Geometry: final body of the model. Coordinates: model frame, mm. Coordinates: 2 decimals unless noted, no trailing zeros. Order: outer loops, then holes, each group sorted by start corner. A loop starts at its lowest first (then second) coordinate and runs counter-clockwise, first axis right, second up. Notation, with made-up numbers: (5.5, 77.25) - (31.5, 77.25) arc R21 ccw to (31.5, 95.25) - close; hole circle Ø3 at (23.5, 72.25). An arc over 180 degrees is marked (long way). Use a Markdown table: item, result. Add a question column.
```python
from build123d import *

# Parameters (mm, degrees)
DOME1_FACE_RADIUS = 41.275
DOME1_HEIGHT      = 9.525
FILLET1_R         = 2.54


# Read off the part's stored shape, not the designer's step: Shell1
with BuildPart() as part:
    # Sketch1 → Revolve1 (revolve)
    with BuildSketch(Plane(origin=(0, 0, 0), x_dir=(0, 0, -1), z_dir=(1, 0, 0)), mode=Mode.PRIVATE) as revolve1_sk:
        Polygon((0, 0), (41.275, 0), (43.78974535, 19.05), (0, 19.05), align=None)
    revolve(revolve1_sk.sketch.rotate(Axis((0, 0, 0), (0, -1, 0)), 180), axis=Axis((0, 0, 0), (0, -1, 0)))

    # Dome1: a dome of height H over a round flat face of radius A is a cap of a sphere of radius (A * A + H * H) / (2 * H)
    dome1_r = (DOME1_FACE_RADIUS * DOME1_FACE_RADIUS + DOME1_HEIGHT * DOME1_HEIGHT) / (2 * DOME1_HEIGHT)
    dome1_base = Plane((0, 0, 0), z_dir=(0, -1, 0))
    with Locations(dome1_base.offset(DOME1_HEIGHT - dome1_r)):
        dome1_ball = Sphere(dome1_r, mode=Mode.PRIVATE)
    add(split(dome1_ball, bisect_by=dome1_base, keep=Keep.TOP, mode=Mode.PRIVATE))

    # Fillet1
    fillet1_edges = [part.edges().sort_by_distance(p)[0] for p in [
        (41.275, 0, 0),
    ]]
    fillet(fillet1_edges, radius=FILLET1_R)

    # Shell1 outline → Shell1 (revolve, cut)
    with BuildSketch(Plane.XY):
        with BuildLine():
            Line((0, 19.05), (0, -6.35))
            ThreePointArc((0, -6.35), (19.639142672, -4.205925769), (38.353009101, 2.125281265))
            Line((38.353009101, 2.125281265), (40.587201031, 19.05))
            Line((40.587201031, 19.05), (0, 19.05))
        make_face()
    revolve(axis=Axis((0, 0, 0), (0, 1, 0)), mode=Mode.SUBTRACT)


solid = part.part
```
1) Section B-B (y = 17). Return loops of the section in (x, z).
2) Pin query (flat end, axial travel): pin 1 (5 mm diameter, centred on x = -33.5, y = 9.5, fed in from +Z); pin 2 (8 mm diameter, centred on x = -30, y = 2.5, fed in from -Z); pin 3 (10 mm diameter, centred on x = -34.5, z = -11.5, fed in from -Y). Return the tip coordinate at first contact, or that it passes through.
3) Section A-A (y = 12.5). Return loops of the section in (x, z), then the cut area to 3 significant figures.
4) Ray query, line 1 along X through (y, z) = (2.75, 19.5); line 2 along X through (y, z) = (12, 9); line 3 along Z through (x, y) = (-7.5, 11). Return the intervals inside material, ascending.
5) Draft query along Z for faces 1 (the face through (40.865, 4.436, -9.075)), 2 (the face through (39, 19.05, 13)), 3 (the face through (36.95, 5.06, -11.64)). Return one class per face: pulls with the +Z half, pulls with the -Z half, needs draft (parallel to the pull), parting line crosses it, or undercut.
Values follow:
| question | item | result |
|---|---|---|
| 1 | outline | circle Ø87.04 at (0, 0); hole circle Ø80.63 at (0, 0) |
| 2 | pin 1 | stops at z = 29.16 |
| 2 | pin 2 | stops at z = -32.55 |
| 2 | pin 3 | stops at y = -4.15 |
| 3 | outline | circle Ø85.85 at (0, 0); hole circle Ø79.45 at (0, 0) |
| 3 | area | 832 mm² |
| 4 | line 1 | x = -36.79 to -33.12, 33.12 to 36.79 |
| 4 | line 2 | x = -41.9 to -38.62, 38.62 to 41.9 |
| 4 | line 3 | z = -42.06 to -38.81, 38.81 to 42.06 |
| 5 | face 1 | parting line crosses it |
| 5 | face 2 | needs draft |
| 5 | face 3 | undercut |
